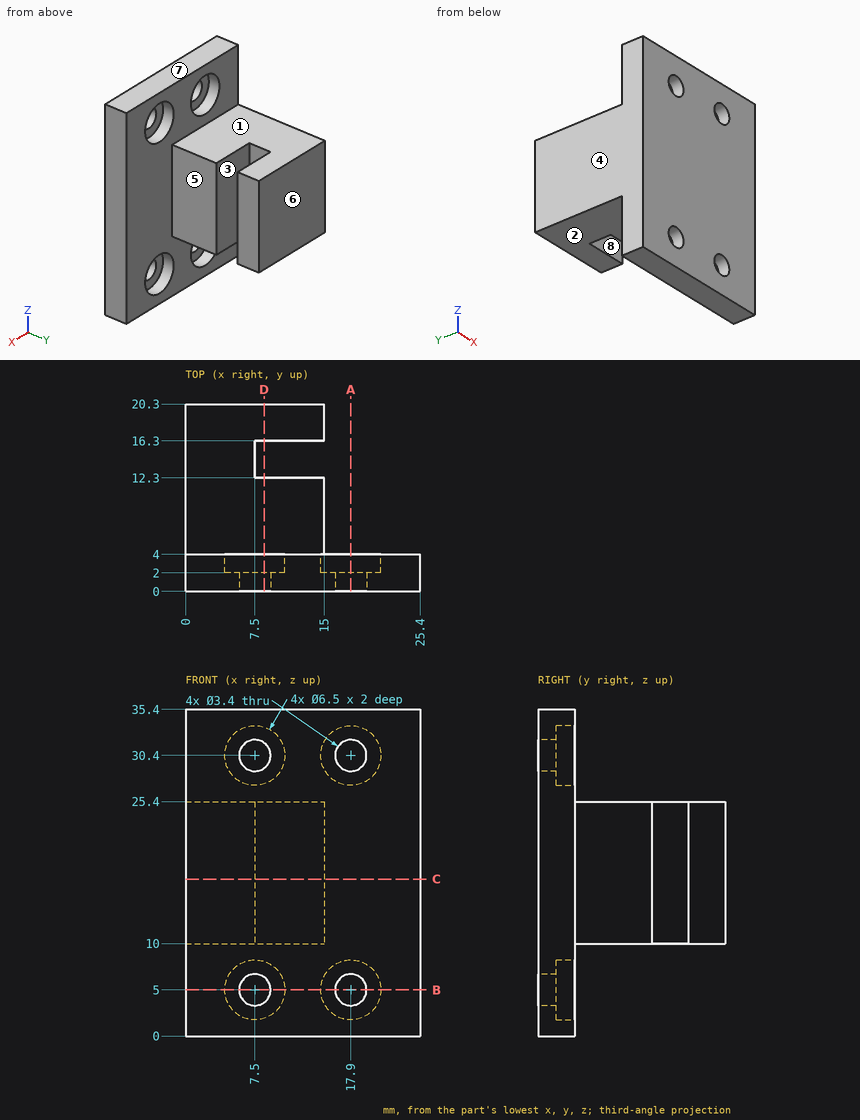
Answer from the drawing. Dimensions are ordinates in mm from the lowest x, y and z of the part. A direction names the side the tool comes from. Round coordinates to 2 decimals unless told otherwise and drop trailing zeros. Order: outer loops, then holes, each group sorted by start corner. A loop starts at its lowest first (then second) coordinate and runs counter-clockwise, first axis right, second up.
1) The part is cut by section A-A on x = 17.9. Write down the section's boundary in (y, z), plus the area to 3 significant figures.
2) The part is cut by section B-B on z = 5. Write down the section's boundary in (x, y).
3) For the marked faces 1, 2, 3, 4 and 5, determine the directions among +Z, -Z, +X, -X, +Y, -Y from which every point of the face is accessible in a straight line to the end or side of a thin tool.
4) The part is cut by section D-D on x = 8.5. Write down the section's boundary in (y, z), plus the area to 3 significant figures.
5) Straight lines are drawn through the part: L1, parallel to X at y = 3.3, z = 30.4; L2, parallel to Z at x = 17.9, y = 0.9; L3, parallel to X at y = 1.5, z = 5. For each, find the intervals that lie inside material, in ascending order.
6) The mould has two halves that part along Y. Classify the marked faces 6, 7 and 8: released by +Y, released by -Y, zero draft, split by the parting line, or undercut.
7) Flat-ended cylindrical pins translate along their axes: pin 1 (5 mm diameter, centred on x = 15, y = 10, fed in from -Z); pin 2 (9 mm diameter, centred on y = 7, z = 21.5, fed in from +X); pin 3 (3 mm diameter, centred on y = 7, z = 4, fed in from -X); pin 4 (7.5 mm diameter, centred on x = 17.9, z = 30.4, fed in from +Y). Find the tip coordinate at first contact, or state that the pin passes through.
8) The part is cut by section C-C on z = 17. Write down the section's boundary in (x, y).
Resolved:
1. outline: (0, 0) - (4, 0) - (4, 1.75) - (2, 1.75) - (2, 3.3) - (0, 3.3) - close; (0, 6.7) - (2, 6.7) - (2, 8.25) - (4, 8.25) - (4, 27.15) - (2, 27.15) - (2, 28.7) - (0, 28.7) - close; (0, 32.1) - (2, 32.1) - (2, 33.65) - (4, 33.65) - (4, 35.4) - (0, 35.4) - close
1. area: 102 mm2
2. outline: (0, 0) - (5.8, 0) - (5.8, 2) - (4.25, 2) - (4.25, 4) - (0, 4) - close; (9.2, 0) - (16.2, 0) - (16.2, 2) - (14.65, 2) - (14.65, 4) - (10.75, 4) - (10.75, 2) - (9.2, 2) - close; (19.6, 0) - (25.4, 0) - (25.4, 4) - (21.15, 4) - (21.15, 2) - (19.6, 2) - close
3. face 1: +Z, +X, -X, +Y
3. face 2: -Z, +X, -X, +Y
3. face 3: +Z, -Z, +X
3. face 4: +Z, -Z, -X, +Y, -Y
3. face 5: +Z, -Z, +X, +Y
4. outline: (0, 0) - (4, 0) - (4, 1.91) - (2, 1.91) - (2, 3.63) - (0, 3.63) - close; (0, 6.37) - (2, 6.37) - (2, 8.09) - (4, 8.09) - (4, 10) - (12.3, 10) - (12.3, 25.4) - (4, 25.4) - (4, 27.31) - (2, 27.31) - (2, 29.03) - (0, 29.03) - close; (0, 31.77) - (2, 31.77) - (2, 33.49) - (4, 33.49) - (4, 35.4) - (0, 35.4) - close; (16.3, 10) - (20.3, 10) - (20.3, 25.4) - (16.3, 25.4) - close
4. area: 295 mm2
5. L1: x = 0 to 4.25, 10.75 to 14.65, 21.15 to 25.4
5. L2: z = 0 to 3.3, 6.7 to 28.7, 32.1 to 35.4
5. L3: x = 0 to 5.8, 9.2 to 16.2, 19.6 to 25.4
6. face 6: released by +Y
6. face 7: zero draft
6. face 8: undercut
7. pin 1: stops at z = 10
7. pin 2: stops at x = 25.4
7. pin 3: passes through
7. pin 4: stops at y = 4
8. outline: (0, 0) - (25.4, 0) - (25.4, 4) - (15, 4) - (15, 12.3) - (7.5, 12.3) - (7.5, 16.3) - (15, 16.3) - (15, 20.3) - (0, 20.3) - close
